Check sheet for the modelled part. Datum: model origin and axes. Units: mm. A direction names the side the tool comes from. Give positions to 0.01 mm unless a question says otherwise; leave off trailing zeros. Loops run counter-clockwise (first coordinate to the right, second up) from the corner with the lowest first, then second, coordinate; pieces in that order, holes last. Notation, with made-up numbers: (7.5, -17.5) - (26.5, -17.5) arc R10 cw to (26.5, -2.5) - close; hole circle Ø1 at (36, -15). An arc over 180 degrees is marked (long way). Use CSV: the item, a comma, the result in double quotes.
Autodesk Inventor part; units mm, degrees
ref_plane "Work Plane1" through (0, 5, 0) normal (1, 0, 0) x (0, 1, 0)
ref_plane "Work Plane2" through (-57.7435, -145.5, 75) normal (0.7434, -0.6689, 0) x (0.6689, 0.7434, 0)
ref_plane "YZ Plane" through (0, 0, 0) normal (1, 0, 0) x (0, 1, 0)
sketch "Sketch1" plane through (0, 0, 0) normal (0, 0, 1) x (1, 0, 0)
  line L0 (0, 0) -> (-50, 0)
  line L1 (-50, 0) -> (-50, 5)
  line L2 (-50, 5) -> (0, 5)
  line L3 (0, 5) -> (0, 0)
  dimension "d0" = 50
  dimension "d1" = 5
extrude "Extrusion1" add sketch "Sketch1" along normal blind 75
sketch "Sketch2" plane through (0, 0, 75) normal (0, 0, 1) x (1, 0, 0)
  circle A0 centre (-225, 5) radius 225 construction
  circle A1 centre (-225, 5) radius 220 construction
  line L0 (0, 0) -> (0, 5)
  line L1 (0, 5) -> (-5, 5)
  arc A2 (-57.7435, -145.5) -> (0, 5) centre (-225, 5) ccw
  line L2 (-57.7435, -145.5) -> (-61.4603, -142.1556)
  arc A3 (-61.4603, -142.1556) -> (-5, 5) centre (-225, 5) ccw
  dimension "d4" = 450
  dimension "d5" = 5
  dimension "d6" = 5
  dimension "d7" = 150.5
extrude "Extrusion2" add sketch "Sketch2" against normal blind 75
sketch "Sketch3" plane through (-50, 5, 0) normal (0, 1, 0) x (1, 0, 0)
  line L0 (45, -10) -> (5, -10)
  line L1 (5, -10) -> (5, -12)
  line L2 (5, -12) -> (45, -12)
  line L3 (45, -12) -> (45, -10)
  line L4 (0, 0) -> (0, -75)
  line L5 (0, 0) -> (50, 0)
  line L6 (5, -17) -> (45, -17)
  line L7 (45, -17) -> (45, -15)
  line L8 (45, -15) -> (5, -15)
  line L9 (5, -15) -> (5, -17)
  line L10 (5, -22) -> (45, -22)
  line L11 (45, -22) -> (45, -20)
  line L12 (45, -20) -> (5, -20)
  line L13 (5, -20) -> (5, -22)
  dimension "d10" = 40
  dimension "d11" = 2
  dimension "d12" = 5
  dimension "d13" = 10
  dimension "d16" = 5
extrude "Extrusion3" cut sketch "Sketch3" against normal blind 5
ref_plane "Work Plane1" through (0, 5, 0) normal (1, 0, 0) x (0, 1, 0)
sketch "Sketch4" plane through (0, 5, 0) normal (1, 0, 0) x (0, 1, 0)
  circle A0 centre (-29.5, 47.5) radius 3
  circle A1 centre (-29.5, 27.5) radius 3
  line L0 (-5, 0) -> (-5, 75)
  line L1 (-150.5, 0) -> (-5, 0)
  circle A2 centre (-39.5, 47.5) radius 3
  circle A3 centre (-39.5, 27.5) radius 3
  line L2 (0, 0) -> (0, 75)
  dimension "d23" = 6
  dimension "d24" = 6
  dimension "d26" = 27.5
  dimension "d27" = 20
  dimension "d30" = 6
  dimension "d31" = 6
  dimension "d32" = 10
  dimension "d33" = 29.5
extrude "Extrusion4" cut sketch "Sketch4" along normal through all both and the other way through all
ref_plane "Work Plane2" through (-57.7435, -145.5, 75) normal (0.7434, -0.6689, 0) x (0.6689, 0.7434, 0)
sketch "Sketch5" plane through (-57.7435, -145.5, 75) normal (0.7434, -0.6689, 0) x (0.6689, 0.7434, 0)
  circle A0 centre (5, -27.5) radius 3
  circle A1 centre (5, -47.5) radius 3
  line L0 (0, 0) -> (0, -75)
  line L1 (0, -75) -> (146.746, -75)
  point P0 (146.7832, -75)
  dimension "d34" = 6
  dimension "d35" = 6
  dimension "d36" = 5
  dimension "d37" = 27.5
  dimension "d38" = 20
extrude "Extrusion5" cut sketch "Sketch5" along normal through all both and the other way through all
sketch "Sketch6" plane through (-50, 0, 0) normal (-1, 0, 0) x (0, 0, 1)
  circle A0 centre (47.5, 2.5) radius 1
  circle A1 centre (27.5, 2.5) radius 1
  line L0 (0, 0) -> (0, 5)
  line L1 (0, 5) -> (75, 5)
  dimension "d41" = 2
  dimension "d42" = 2
  dimension "d43" = 27.5
  dimension "d44" = 20
  dimension "d45" = 2.5
extrude "Extrusion6" cut sketch "Sketch6" against normal blind 10
thread "Thread1"
thread "Thread2"
sketch "Sketch7" plane through (0, 0, 75) normal (0, 0, 1) x (1, 0, 0)
  circle A0 centre (-225, 5) radius 225
  circle A1 centre (-225, 5) radius 230
  point P0 (0, 0)
  point P1 (0, 5)
  dimension "d52" = 450
  dimension "d53" = 5
extrude "Extrusion7" cut sketch "Sketch7" against normal through all
properties part number "CW005" material "ABS Plastic"
1. Set-up check for faces 1 (the face through (-50, 2, 37)), 2 (the face through (-55.21, -138.88, 50.03)), 3 (the face through (-25, 3, 15)), 4 (the face through (-20.914, -77.152, 38.025)): record each of +Z, -Z, +X, -X, +Y, -Y from which the full face is reachable in a straight line by a thin tool's end or side.
Completed:
face 1,"+Z, -Z, -X, +Y"
face 2,"none"
face 3,"+Y"
face 4,"+Z, -Z, -X"
2. Sectioned sample at B-B, the plane y = -34.5. Record the boundary of the cut face in (x, z).
Completed:
outline,"(-8.58, 0) - (-3.49, 0) - (-3.49, 24.5) - (-8.58, 24.5) - close; (-8.58, 30.5) - (-3.49, 30.5) - (-3.49, 44.5) - (-8.58, 44.5) - close; (-8.58, 50.5) - (-3.49, 50.5) - (-3.49, 75) - (-8.58, 75) - close"
3. Sectioned sample at C-C, the plane z = 68. Record the boundary of the cut face in (x, y).
Completed:
outline,"(-61.46, -142.16) - (-57.74, -145.5) arc R225 ccw to (-0.06, 0) arc R225 ccw to (0, 5) - (-50, 5) - (-50, 0) - (-5.06, 0) arc R220 cw to start"
4. Release check for a two-part mould opening along Z. For faces 5 (the face through (-13, -59, 0)), 6 (the face through (-27, 0, 45)), 7 (the face through (-4.45, -25.15, 44.57)), 8 (the face through (-6.019, -33.116, 24.838)) record: released by +Z, released by -Z, zero draft, split by the parting line, or undercut.
Completed:
face 5,"released by -Z"
face 6,"zero draft"
face 7,"undercut"
face 8,"undercut"
5. Go/stop test with flat-tipped pins: pin 1 Ø5 at (y, z) = (-34.5, 47.5) entering from +X; pin 2 Ø1.5 at (y, z) = (2.5, 53) entering from -X; pin 3 Ø6 at (y, z) = (-63, 58) entering from -X; pin 4 Ø3 at (y, z) = (-118, 46.5) entering from +X. Record where each tip stops, or that it passes through.
Completed:
pin 1,"passes through"
pin 2,"stops at x = -50"
pin 3,"stops at x = -16.77"
pin 4,"stops at x = -35.63"
6. Sectioned sample at D-D, the plane y = -133.5. Record the boundary of the cut face in (x, z), and give its area (3 significant figures).
Completed:
outline,"(-54.07, 0) - (-47.68, 0) - (-47.68, 75) - (-54.07, 75) - close"
area,"479 mm²"
7. Sectioned sample at A-A, the plane x = -12.5. Record the boundary of the cut face in (y, z), and give its area (3 significant figures).
Completed:
outline,"(-68.95, 0) - (-51.95, 0) - (-51.95, 75) - (-68.95, 75) - close; (0, 0) - (5, 0) - (5, 10) - (0, 10) - close; (0, 12) - (5, 12) - (5, 15) - (0, 15) - close; (0, 17) - (5, 17) - (5, 20) - (0, 20) - close; (0, 22) - (5, 22) - (5, 75) - (0, 75) - close"
area,"1,620 mm²"
8. Scan lines: line 1 along Z through (x, y) = (-6, -34); line 2 along Y through (x, z) = (-42, 27); line 3 along Y through (x, z) = (-43.5, 27). Record each from-to range of solid material in increasing order.
Completed:
line 1,"z = 0 to 24.54, 30.46 to 44.54, 50.46 to 75"
line 2,"y = -125.9 to -117.11, 0 to 1.63, 3.37 to 5"
line 3,"y = -127.98 to -119.33, 0 to 1.63, 3.37 to 5"
